Here's the drawing with two shaded views (mm, measured from the low corner). I have some questions. Round coordinates to 2 decimals unless told otherwise and drop trailing zeros. Loops run counter-clockwise (first coordinate to the right, second up) from the corner with the lowest first, then second, coordinate; pieces in that order, holes last. Notation, with made-up numbers: M 89.5,15.5 L 133.5,15.5 A11 ccw 133.5,33.5 Z; hole C 54,82 d6. An arc over 180 degrees is marked long. One line per item, written item: value. Start each with the question number.
Q1. Imagine slicing it at C-C (y = 1.5). Please give me the cut outline in (x, z), then the cut area to 3 significant figures.
Q2. Please list where these lines run through material, in increasing order: line 1 along Z through (x, y) = (9.5, 1.2); line 2 along Z through (x, y) = (7.25, 0.75); line 3 along Z through (x, y) = (9, 0.95).
Q3. Imagine slicing it at D-D (x = 16.25). Please give me the cut outline in (y, z).
Q4. I'm going to push flat-ended pins straight in: pin 1 Ø2.5 at (x, z) = (9.5, 3.5) entering from -Y; pin 2 Ø1 at (x, y) = (6.5, 2.5) entering from +Z; pin 3 Ø2.5 at (x, z) = (2.5, 9.5) entering from +Y. Where does each tip first touch, or does it pass through?
Q5. Thinking about a two-plate mould opening in X: for the marked faces 1, 2 and 3, which applies, released by +X, released by -X, zero draft, split by the parting line, or undercut?
Q6. Imagine slicing it at A-A (x = 9.5). Give the number of separate pieces and of enclosed holes in the cut face, then the cut area to 3 significant figures.
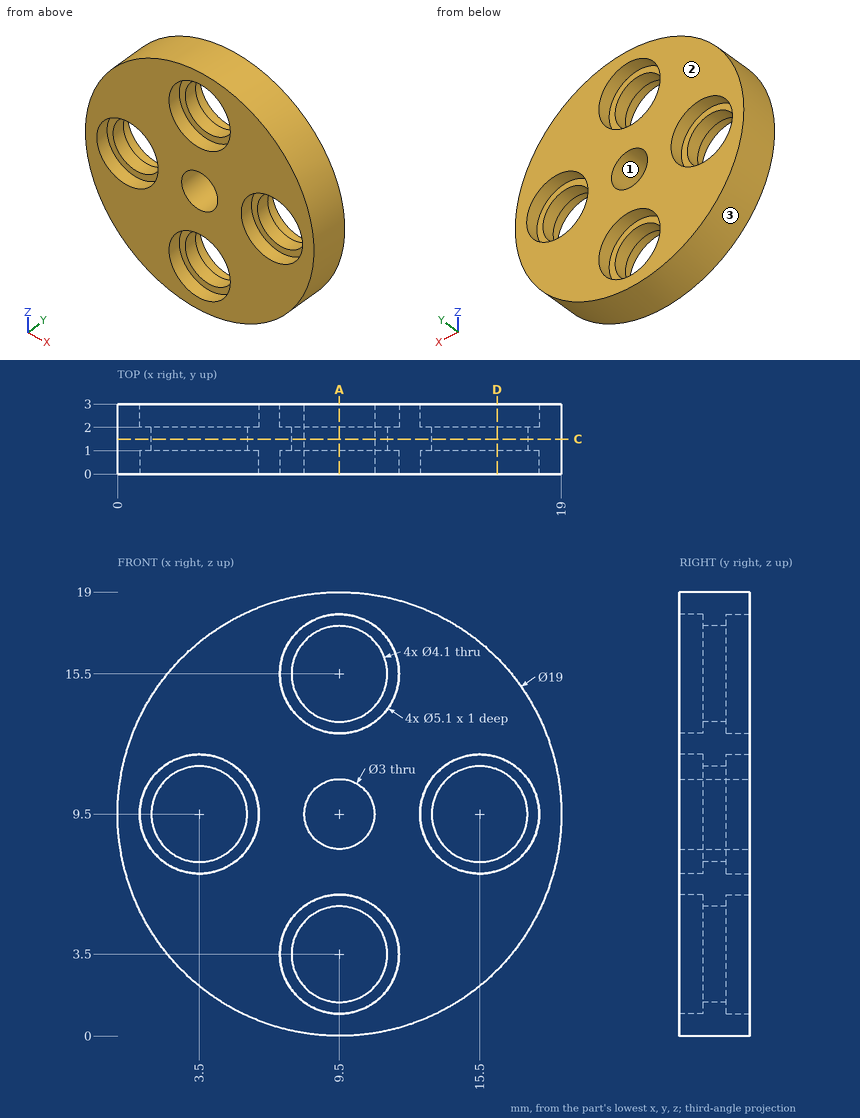
Report:
1. outline: C 9.5,9.5 d19; hole C 3.5,9.5 d4.1; hole C 9.5,3.5 d4.1; hole C 9.5,15.5 d4.1; hole C 9.5,9.5 d3; hole C 15.5,9.5 d4.1
1. area: 224 mm²
2. line 1: z = 0 to 1.45, 5.55 to 8, 11 to 13.45, 17.55 to 19
2. line 2: z = 0.27 to 2.3, 4.7 to 14.3, 16.7 to 18.73
2. line 3: z = 0.01 to 1, 6 to 8.09, 10.91 to 13, 18 to 18.99
3. outline: M 0,2.82 L 3,2.82 L 3,7.06 L 2,7.06 L 2,7.59 L 1,7.59 L 1,7.06 L 0,7.06 Z; M 0,11.94 L 1,11.94 L 1,11.41 L 2,11.41 L 2,11.94 L 3,11.94 L 3,16.18 L 0,16.18 Z
4. pin 1: passes through
4. pin 2: stops at z = 18.67
4. pin 3: stops at y = 2
5. face 1: undercut
5. face 2: zero draft
5. face 3: split by the parting line
6. separate pieces: 4
6. enclosed holes: 0
6. area: 19.4 mm²
